Can you work these out from the model? Positions are in its coordinate system, mm. A direction names the side the tool comes from. Give positions to 0.01 mm unless a question says otherwise; leave off trailing zeros. Write each loop counter-clockwise with the first axis right and the second up, starting at its lowest first coordinate (ties: lowest second). Pieces come first, ordered by that corner, then holes. Notation, with made-up numbers: (-33.75, -30) -> (-8.75, -30) arc R31 ccw to (-8.75, 7) -> close; hole circle Ø9 at (42, 46.25). An arc over 180 degrees is marked (long way). One line per item, written item: value.
from build123d import *

# Parameters (mm, degrees)
SKETCH1_R           = 17.4
BOSS_EXTRUDE1_DEPTH = 15.4
SKETCH6_R           = 17
BOSS_EXTRUDE5_DEPTH = 30.7
SKETCH7_R           = 18.4
BOSS_EXTRUDE6_DEPTH = 20
SKETCH2_R           = 6
BOSS_EXTRUDE2_DEPTH = 6
SKETCH3_R           = 3
BOSS_EXTRUDE4_DEPTH = 10
SKETCH4_W           = 6
SKETCH4_H           = 8
CUT_EXTRUDE1_DEPTH  = 10
BOSS_EXTRUDE7_DEPTH = 1
SKETCH5_R           = 1.5
CUT_EXTRUDE2_DEPTH  = 3


with BuildPart() as part:
    # Sketch1 → Boss-Extrude1 (new body)
    with BuildSketch(Plane(origin=(0, 0, 0), x_dir=(1, 0, 0), z_dir=(0, 1, 0))):
        with Locations(Location((0, 0, 0), (0, 0, 90))):
            Circle(SKETCH1_R)
    extrude(amount=BOSS_EXTRUDE1_DEPTH)

    # Sketch6 → Boss-Extrude5 (add)
    with BuildSketch(Plane(origin=(0, 15.4, 0), x_dir=(1, 0, 0), z_dir=(0, 1, 0))):
        with Locations(Location((0, 0, 0), (0, 0, 270))):
            Circle(SKETCH6_R)
    extrude(amount=BOSS_EXTRUDE5_DEPTH)

    # Sketch7 → Boss-Extrude6 (add)
    with BuildSketch(Plane(origin=(0, 46.1, 0), x_dir=(1, 0, 0), z_dir=(0, 1, 0))):
        with Locations(Location((0, 0, 0), (0, 0, 270))):
            Circle(SKETCH7_R)
    extrude(amount=BOSS_EXTRUDE6_DEPTH)

    # Sketch2 → Boss-Extrude2 (add)
    with BuildSketch(Plane(origin=(0, 66.1, 0), x_dir=(1, 0, 0), z_dir=(0, 1, 0))):
        with Locations(Location((0, -7, 0), (0, 0, 270))):
            Circle(SKETCH2_R)
    extrude(amount=BOSS_EXTRUDE2_DEPTH)

    # Sketch3 → Boss-Extrude4 (add)
    with BuildSketch(Plane(origin=(0, 72.1, 0), x_dir=(1, 0, 0), z_dir=(0, 1, 0))):
        with Locations(Location((0, -7, 0), (0, 0, 270))):
            Circle(SKETCH3_R)
    extrude(amount=BOSS_EXTRUDE4_DEPTH)

    # Sketch4 → Cut-Extrude1 (cut)
    with BuildSketch(Plane.XY.offset(4.6)):
        with Locations((0, 78.1)):
            Rectangle(SKETCH4_W, SKETCH4_H)
    extrude(amount=-CUT_EXTRUDE1_DEPTH, mode=Mode.SUBTRACT)

    # Sketch8 → Boss-Extrude7 (add)
    with BuildSketch(Plane.XZ.offset(-15.4)):
        Polygon((2.828427125, -2.828427125), (-2.828427125, 2.828427125), (12.727922061, 18.384776311), (18.384776311, 12.727922061), align=None)
    extrude(amount=BOSS_EXTRUDE7_DEPTH)

    # Sketch5 → Cut-Extrude2 (cut)
    with BuildSketch(Plane(origin=(0, 66.1, 0), x_dir=(1, 0, 0), z_dir=(0, 1, 0))):
        with Locations(Location((-7.75, 13.423393759, 0), (0, 0, 270))):
            Circle(SKETCH5_R)
        with Locations(Location((7.75, 13.423393759, 0), (0, 0, 270))):
            Circle(SKETCH5_R)
        with Locations(Location((-15.5, 0, 0), (0, 0, 270))):
            Circle(SKETCH5_R)
        with Locations(Location((15.5, 0, 0), (0, 0, 270))):
            Circle(SKETCH5_R)
        with Locations(Location((7.75, -13.423393759, 0), (0, 0, 270))):
            Circle(SKETCH5_R)
        with Locations(Location((-7.75, -13.423393759, 0), (0, 0, 270))):
            Circle(SKETCH5_R)
    extrude(amount=-CUT_EXTRUDE2_DEPTH, mode=Mode.SUBTRACT)


solid = part.part
1) If we section it at C-C (z = 0): Write out the boundary of the cut face in (x, y), and give its area (3 significant figures).
Answer list:
outline: (-18.4, 46.1) -> (-17, 46.1) -> (-17, 15.4) -> (-17.4, 15.4) -> (-17.4, 0) -> (17.4, 0) -> (17.4, 15.4) -> (17, 15.4) -> (17, 46.1) -> (18.4, 46.1) -> (18.4, 66.1) -> (17, 66.1) -> (17, 63.1) -> (14, 63.1) -> (14, 66.1) -> (-14, 66.1) -> (-14, 63.1) -> (-17, 63.1) -> (-17, 66.1) -> (-18.4, 66.1) -> close
area: 2,300 mm^2
2) If we section it at D-D (y = 52.5): Write out the boundary of the cut face in (x, z), and give its area (3 significant figures).
Answer list:
outline: circle Ø36.8 at (0, 0)
area: 1,060 mm^2
3) Will these pins go through, and if not, where does the flat tip stop? pin 1 (5 mm diameter, centred on x = -12, z = -12, fed in from +Y); pin 2 (2.5 mm diameter, centred on x = 7.75, z = 13.42, fed in from +Y); pin 3 (3 mm diameter, centred on x = 13, z = 14, fed in from -Y).
Answer list:
pin 1: stops at y = 66.1
pin 2: stops at y = 63.1
pin 3: stops at y = 14.4
4) For faces 1 (the face through (14, 14.4, 14)), 2 (the face through (16.619, 14.907, 10.962)), 3 (the face through (-9.214, 64.621, -13.749)), 4 (the face through (-5.226, 7.592, -16.597)), 5 (the face through (12, 15.4, 13)), which set-ups out of +Z, -Z, +X, -X, +Y, -Y let a thin tool reach every point of the face, with its end or its side?
Answer list:
face 1: +Z, +X, -Y
face 2: +X, -Y
face 3: +Y
face 4: -Y
face 5: none
5) If we section it at A-A (x = 0): Write out the boundary of the cut face in (y, z).
Answer list:
outline: (0, -17.4) -> (15.4, -17.4) -> (15.4, -17) -> (46.1, -17) -> (46.1, -18.4) -> (66.1, -18.4) -> (66.1, 1) -> (72.1, 1) -> (72.1, 4) -> (74.1, 4) -> (74.1, 4.6) -> (82.1, 4.6) -> (82.1, 10) -> (72.1, 10) -> (72.1, 13) -> (66.1, 13) -> (66.1, 18.4) -> (46.1, 18.4) -> (46.1, 17) -> (15.4, 17) -> (15.4, 17.4) -> (0, 17.4) -> close
6) If we section it at B-B (y = 64): Write out the boundary of the cut face in (x, z).
Answer list:
outline: circle Ø36.8 at (0, 0); hole circle Ø3 at (-15.5, 0); hole circle Ø3 at (-7.75, -13.42); hole circle Ø3 at (-7.75, 13.42); hole circle Ø3 at (7.75, -13.42); hole circle Ø3 at (7.75, 13.42); hole circle Ø3 at (15.5, 0)
7) I need wall thicknesses on L1, parallel to X at y = 65.3, z = 0; L2, parallel to Z at x = 0, y = 29; L3, parallel to Y at x = 8.5, z = -9. Which ranges of each line are inside material? Lowest first, please.
Answer list:
L1: x = -18.4 to -17, -14 to 14, 17 to 18.4
L2: z = -17 to 17
L3: y = 0 to 66.1
8) We'd pull the mould along Z, two halves only. Please class faces 6 (the face through (0, 78, 4.6)), 7 (the face through (16.855, 30.535, -2.213)), 8 (the face through (-8, 63.1, 13)): released by +Z, released by -Z, zero draft, split by the parting line, or undercut.
Answer list:
face 6: released by -Z
face 7: split by the parting line
face 8: undercut
